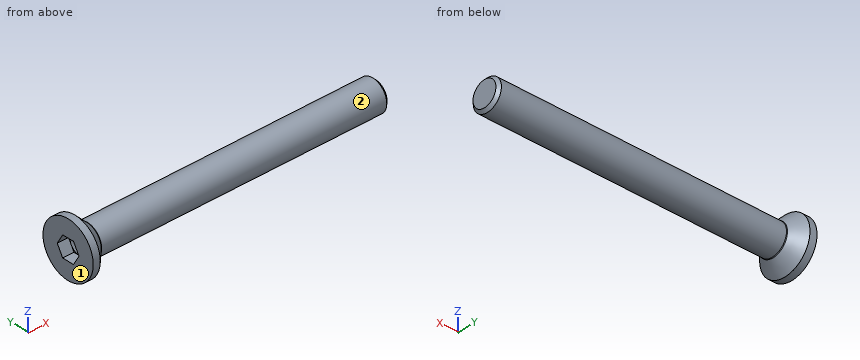
```python
from build123d import *

# Parameters (mm, degrees)
FILLET1_R   = 0.1
HEX_START   = -1.1
HEX_2_DEPTH = 1.1


with BuildPart() as part:
    # BodySke → BaseBody (revolve)
    with BuildSketch(Plane.XY, mode=Mode.PRIVATE) as basebody_sk:
        Polygon((0, 0), (0, 2.675), (0.685, 2.675), (1.86, 1.5), (29.7195, 1.5), (30, 1.2195), (30, 0), align=None)
    revolve(basebody_sk.sketch.rotate(Axis((0, 0, 0), (1, 0, 0)), 90), axis=Axis((0, 0, 0), (1, 0, 0)))

    # Fillet1
    fillet1_edges = [part.edges().sort_by_distance(p)[0] for p in [
        (1.86, 0, -1.5),
    ]]
    fillet(fillet1_edges, radius=FILLET1_R)

    # Hex 2: read off the stored shape, not the designer's step
    # Hex 2 outline → Hex 2 (cut)
    with BuildSketch(Plane.ZY.offset(HEX_START)):
        Polygon((-1, -0.577350269), (0, -1.154700538), (1, -0.577350269), (1, 0.577350269), (0, 1.154700538), (-1, 0.577350269), align=None)
    extrude(amount=HEX_2_DEPTH, mode=Mode.SUBTRACT)

    # Hex 2 2 outline → Hex 2 2 (revolve, cut)
    with BuildSketch(Plane.YX):
        Polygon((1, 1.1), (0, 1.677350269), (0, 1.1), align=None)
    revolve(axis=Axis((0, 0, 0), (1, 0, 0)), mode=Mode.SUBTRACT)


solid = part.part
```
The listing builds one solid part. Answer for the finished solid, in the listing's coordinates (mm). Face numbers are marked on the shaded views. A direction names the side the tool comes from. Coordinates: 2 decimals unless noted, no trailing zeros. Write each loop counter-clockwise with the first axis right and the second up, starting at its lowest first coordinate (ties: lowest second). Pieces come first, ordered by that corner, then holes.
Q1. Find the intervals of material crossed by line 1 along X through (y, z) = (-0.3, -1.8); line 2 along X through (y, z) = (-0.1, -2.35); line 3 along Z through (x, y) = (23.25, 0.05), in increasing order.
Returned:
line 1: x = 0 to 1.54
line 2: x = 0 to 1.01
line 3: z = -1.5 to 1.5
Q2. Given P1, Ø3, axis at x = 25, y = -1, coming from the -Z side; P2, Ø1.5, axis at y = -0.5, z = 2, coming from the +X side; P3, Ø2, axis at x = 14, y = -1.5, coming from the -Z side, each flat-ended and moving along its own axis, determine where each tip first touches the part or whether it passes through.
Returned:
P1: stops at z = -1.5
P2: stops at x = 29.91
P3: stops at z = -1.41
Q3. Section A-A, the plane x = 12.25 is taken. Write down the section's boundary in (y, z), then the cut area to 3 significant figures.
Returned:
outline: circle Ø3 at (0, 0)
area: 7.07 mm2
Q4. Which of the six approach directions +Z, -Z, +X, -X, +Y, -Y give full straight-line access (tool end or side, diameter ignored) to the marked faces 1 and 2?
Returned:
face 1: +Z, -Z, -X, +Y, -Y
face 2: +X
